Design review of the part built by this model. Coordinates are the model's own, in mm. A direction names the side the tool comes from. Coordinates: 2 decimals unless noted, no trailing zeros. Write each loop counter-clockwise with the first axis right and the second up, starting at its lowest first coordinate (ties: lowest second). Pieces come first, ordered by that corner, then holes. Notation, with made-up numbers: (63, 26.5) - (109, 26.5) arc R30 cw to (109, 49.5) - close; hole circle Ø1 at (53.5, -39.5). An arc over 180 degrees is marked (long way). Answer as CSV lines item,"result". Start each with the question number.
Q1. We need section D-D (z = 52.5). Write out the cut boundary in (x, y).
Q2. Mouldability with a two-part tool opening along Z and no side actions: class faces 3 (the face through (-2, -7, 70)), 4 (the face through (8.1, -0.7, -55.5)), 5 (the face through (24, 0, -1)), 6 (the face through (-99.93, -0.74, 51.85)) as pulls with the +Z half, pulls with the -Z half, needs draft (parallel to the pull), parting line crosses it, or undercut.
Q3. We need section B-B (y = -8.5). Write out the cut boundary in (x, z).
Q4. We need section A-A (x = 104). Write out the cut boundary in (y, z).
Q5. Clearance check with flat-ended pins moving along their axes: pin 1 (9.5 mm diameter, centred on x = 8, z = -52.5, fed in from -Y); pin 2 (3.5 mm diameter, centred on x = 8, z = 52.5, fed in from -Y). State where each tip first meets the part, or that it passes through.
Q6. Machinability: for faces 1 (the face through (101.9, -0.7, 49.7)), 2 (the face through (24, -1.5, 1)), which of the approach directions +Z, -Z, +X, -X, +Y, -Y give a long, thin tool a straight path to every point of the face, cutting with its end or side? Answer none if there is none.
Q7. We need section C-C (z = 0). Write out the cut boundary in (x, y).
Q8. For line 1 along Z through (x, y) = (-55.5, -7.25); line 2 along X through (y, z) = (-0.6, 52.5); line 3 along Y through (x, z) = (-100, -39), list the stretches that pass through material, from the lowest coordinate up. Write a range as [from, to].
from build123d import *

# Parameters (mm, degrees)
SM_START               = -117
SM_BASE_FLANGE_1_DEPTH = 234
SKETCH_7_R             = 59
SKETCH_7_R_2           = 3
SKETCH_7_R_3           = 3.5
CUT_EXTRUDE_1_DEPTH    = 137.868550076


# Read off the part's stored shape, not the designer's step: 基体-法兰1
with BuildPart() as part:
    # 基体-法兰1 outline → 基体-法兰1 (new body)
    with BuildSketch(Plane(origin=(0, 0, 0), x_dir=(0, 0, -1), z_dir=(1, 0, 0)).offset(SM_START)):
        with BuildLine():
            Line((68.5, -1.5), (68.5, -12))
            Line((68.5, -12), (70, -12))
            Line((70, -12), (70, -1.5))
            ThreePointArc((70, -1.5), (69.560660172, -0.439339828), (68.5, 0))
            Line((68.5, 0), (-68.5, 0))
            ThreePointArc((-68.5, 0), (-69.560660172, -0.439339828), (-70, -1.5))
            Line((-70, -1.5), (-70, -12))
            Line((-70, -12), (-68.5, -12))
            Line((-68.5, -12), (-68.5, -1.5))
            Line((-68.5, -1.5), (68.5, -1.5))
        make_face()
    extrude(amount=SM_BASE_FLANGE_1_DEPTH)

    # 草图7 → 切除-拉伸1 (cut, through all)
    with BuildSketch(Plane(origin=(0, 0, 0), x_dir=(1, 0, 0), z_dir=(0, 1, 0))):
        with Locations(Location((-44.5, 0, 0), (0, 0, 270))):
            Circle(SKETCH_7_R)
        with Locations(Location((-97, 52.5, 0), (0, 0, 270))):
            Circle(SKETCH_7_R_2)
        with Locations(Location((8, 52.5, 0), (0, 0, 270))):
            Circle(SKETCH_7_R_2)
        with Locations(Location((8, -52.5, 0), (0, 0, 270))):
            Circle(SKETCH_7_R_2)
        with Locations(Location((-97, -52.5, 0), (0, 0, 270))):
            Circle(SKETCH_7_R_2)
        with Locations(Location((104, 52.5, 0), (0, 0, 270))):
            Circle(SKETCH_7_R_3)
        with Locations(Location((104, -52.5, 0), (0, 0, 270))):
            Circle(SKETCH_7_R_3)
    extrude(amount=-CUT_EXTRUDE_1_DEPTH, mode=Mode.SUBTRACT)


solid = part.part
Results list:
1,outline,"(-117, -1.5) - (-100, -1.5) - (-100, 0) - (-117, 0) - close; (-94, -1.5) - (-71.42, -1.5) - (-71.42, 0) - (-94, 0) - close; (-17.58, -1.5) - (5, -1.5) - (5, 0) - (-17.58, 0) - close; (11, -1.5) - (100.5, -1.5) - (100.5, 0) - (11, 0) - close; (107.5, -1.5) - (117, -1.5) - (117, 0) - (107.5, 0) - close"
2,face 3,"pulls with the +Z half"
2,face 4,"undercut"
2,face 5,"needs draft"
2,face 6,"undercut"
3,outline,"(-117, -70) - (117, -70) - (117, -68.5) - (-117, -68.5) - close; (-117, 68.5) - (117, 68.5) - (117, 70) - (-117, 70) - close"
4,outline,"(-12, -70) - (-1.5, -70) arc R1.5 ccw to (0, -68.5) - (0, -56) - (-1.5, -56) - (-1.5, -68.5) - (-12, -68.5) - close; (-12, 68.5) - (-1.5, 68.5) - (-1.5, 56) - (0, 56) - (0, 68.5) arc R1.5 ccw to (-1.5, 70) - (-12, 70) - close; (-1.5, -49) - (0, -49) - (0, 49) - (-1.5, 49) - close"
5,pin 1,"stops at y = -1.5"
5,pin 2,"passes through"
6,face 1,"+Y, -Y"
6,face 2,"+X, -X, -Y"
7,outline,"(-117, -1.5) - (-103.5, -1.5) - (-103.5, 0) - (-117, 0) - close; (14.5, -1.5) - (117, -1.5) - (117, 0) - (14.5, 0) - close"
8,line 1,"z = [-70, -68.5], [68.5, 70]"
8,line 2,"x = [-117, -100], [-94, -71.42], [-17.58, 5], [11, 100.5], [107.5, 117]"
8,line 3,"y = [-1.5, 0]"
